Verification items for this drawing (mm, ordinates from the low corner). A direction names the side the tool comes from. Round coordinates to 2 decimals unless told otherwise and drop trailing zeros. Loops run counter-clockwise (first coordinate to the right, second up) from the corner with the lowest first, then second, coordinate; pieces in that order, holes last. Notation, with made-up numbers: (62.5, 48.25) -> (104.5, 48.25) arc R18 ccw to (104.5, 71.25) -> close; hole circle Ø1 at (3, 17.5). An arc over 180 degrees is marked (long way). One line per item, written item: value. Start each with the question number.
1. Cross-section at B-B on x = 85. Record the cut outline in (y, z), then the cut area to 4 significant figures.
2. Cross-section at A-A on z = 27.5. Record the cut outline in (x, y), then the cut area to 3 significant figures.
3. Cross-section at C-C on y = 10. Record the cut outline in (x, z), then the cut area to 3 significant figures.
4. Release check for a two-part mould opening along X. For the marked faces 5, 6, 7 and 8 record: +X half, -X half, draft (parallel to the pull), parting line (faces both ways), or undercut.
5. Material ranges on L1, parallel to X at y = 0.5, z = 2; L2, parallel to Z at x = 85, y = 4.5; L3, parallel to X at y = 1.75, z = 14, recorded low to high.
6. Set-up check for the marked faces 1, 2, 3 and 4: record each of +Z, -Z, +X, -X, +Y, -Y from which the full face is reachable in a straight line by a thin tool's end or side.
7. Go/stop test with flat-tipped pins: pin 1 (3.5 mm diameter, centred on x = 45, z = 5, fed in from -Y); pin 2 (5 mm diameter, centred on x = 24.5, z = 7, fed in from -Y); pin 3 (4 mm diameter, centred on x = 11.5, y = 5, fed in from -Z); pin 4 (4 mm diameter, centred on x = 10, y = 6, fed in from +Z). Record where each tip stops, or that it passes through.
8. Cross-section at D-D on y = 3.5. Count the separate pieces of the cut face and the enclosed holes in it, then the cut area to 3 significant figures.
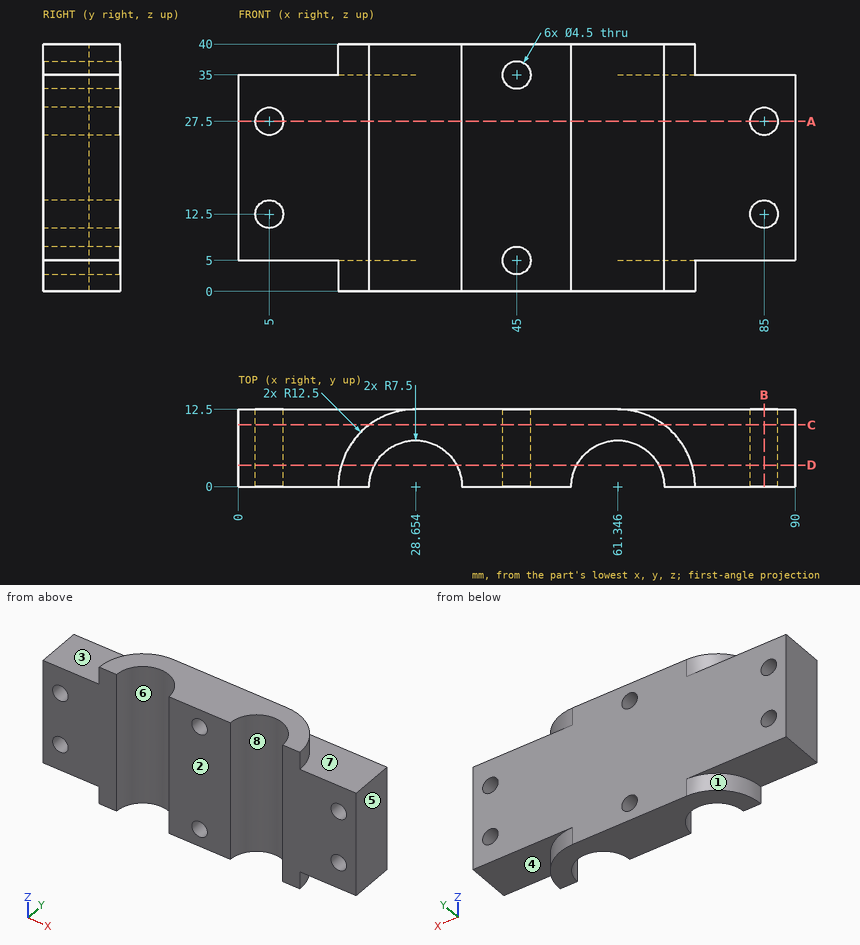
Taken from the geometry:
1. outline: (0, 5) -> (12.5, 5) -> (12.5, 10.25) -> (0, 10.25) -> close; (0, 14.75) -> (12.5, 14.75) -> (12.5, 25.25) -> (0, 25.25) -> close; (0, 29.75) -> (12.5, 29.75) -> (12.5, 35) -> (0, 35) -> close
1. area: 262.5 mm2
2. outline: (0, 0) -> (2.75, 0) -> (2.75, 12.5) -> (0, 12.5) -> close; (7.25, 0) -> (21.15, 0) arc R7.5 cw to (36.15, 0) -> (53.85, 0) arc R7.5 cw to (68.85, 0) -> (82.75, 0) -> (82.75, 12.5) -> (7.25, 12.5) -> close; (87.25, 0) -> (90, 0) -> (90, 12.5) -> (87.25, 12.5) -> close
2. area: 836 mm2
3. outline: (0, 5) -> (21.15, 5) -> (21.15, 0) -> (68.85, 0) -> (68.85, 5) -> (90, 5) -> (90, 35) -> (68.85, 35) -> (68.85, 40) -> (21.15, 40) -> (21.15, 35) -> (0, 35) -> close; hole circle Ø4.5 at (5, 12.5); hole circle Ø4.5 at (5, 27.5); hole circle Ø4.5 at (45, 5); hole circle Ø4.5 at (45, 35); hole circle Ø4.5 at (85, 12.5); hole circle Ø4.5 at (85, 27.5)
3. area: 3,080 mm2
4. face 5: +X half
4. face 6: undercut
4. face 7: draft
4. face 8: undercut
5. L1: x = 16.16 to 21.17, 36.14 to 53.86, 68.83 to 73.84
5. L2: z = 5 to 10.25, 14.75 to 25.25, 29.75 to 35
5. L3: x = 0 to 3.32, 6.68 to 21.36, 35.95 to 54.05, 68.64 to 83.32, 86.68 to 90
6. face 1: -Z, -X, +Y
6. face 2: +Z, -Z, +X, -X, -Y
6. face 3: +Z, -X, +Y
6. face 4: -Z, +X, +Y
7. pin 1: passes through
7. pin 2: stops at y = 3.46
7. pin 3: stops at z = 5
7. pin 4: stops at z = 35
8. separate pieces: 3
8. enclosed holes: 6
8. area: 2,110 mm2
